```python
from build123d import *

# Parameters (mm, degrees)
F0_R     = 28.3
F0_R_2   = 26.5
F1_DEPTH = 8
F2_SIZE  = 1.5
F3_SIZE  = 0.5
F4_R     = 29.8
F4_R_2   = 28.3
F5_DEPTH = 4.5
F6_SIZE  = 1.49999
F7_SIZE  = 0.5


# Not quite as in the source:
# - a fillet or chamfer is up to 0.001 mm smaller than in the source, because OpenCascade refuses the exact size


with BuildPart() as f1:
    # F0 (on Top) → F1 (new body)
    with BuildSketch(Plane.XY):
        Circle(F0_R)
        Circle(F0_R_2, mode=Mode.SUBTRACT)
    extrude(amount=F1_DEPTH)

    # F2
    f2_edges = [f1.edges().sort_by_distance(p)[0] for p in [
        (-28.3, 0, 8),
    ]]
    chamfer(f2_edges, length=F2_SIZE)

    # F3
    f3_edges = [f1.edges().sort_by_distance(p)[0] for p in [
        (-26.5, 0, 0),
    ]]
    chamfer(f3_edges, length=F3_SIZE)

    # F4 (on face) → F5 (join)
    with BuildSketch(Plane(origin=(0, 0, 0), x_dir=(1, 0, 0), z_dir=(0, 0, -1))):
        Circle(F4_R)
        Circle(F4_R_2, mode=Mode.SUBTRACT)
    extrude(amount=-F5_DEPTH)

    # F6 (size 1.5 in the source; OpenCascade refuses exactly that, so slightly less here)
    f6_edges = [f1.edges().sort_by_distance(p)[0] for p in [
        (-29.8, 0, 4.5),
    ]]
    chamfer(f6_edges, length=F6_SIZE)

    # F7
    f7_edges = [f1.edges().sort_by_distance(p)[0] for p in [
        (-29.8, 0, 0),
    ]]
    chamfer(f7_edges, length=F7_SIZE)


solid = f1.part
```
The listing builds one solid part. Answer for the finished solid, in the listing's coordinates (mm). Round coordinates to 2 decimals unless told otherwise and drop trailing zeros. Write each loop counter-clockwise with the first axis right and the second up, starting at its lowest first coordinate (ties: lowest second). Pieces come first, ordered by that corner, then holes. Notation, with made-up numbers: (0.5, 21) -> (23.5, 21) arc R34 ccw to (23.5, 53) -> close; hole circle Ø7 at (12.5, -33.5). An arc over 180 degrees is marked (long way). Use CSV: the item, a comma, the result in double quotes. Start each with the question number.
(1) Section C-C on z = 3.75 is taken. Give the vertices of the cut face in (x, y), then the cut area to 3 significant figures.
(2) Consider L1, parallel to Y at x = 0, z = 3; L2, parallel to Y at x = 0, z = 5.25; L3, parallel to X at y = -14.5, z = 2.75. Determine where each line is inside the solid, lowest interval first. Write a range as from..to.
(3) Each of these flat-tipped pins is pushed along its axis until it touches: pin 1 (1.5 mm diameter, centred on y = 8.5, z = 3, fed in from -X); pin 2 (2 mm diameter, centred on y = -8, z = 6, fed in from -X); pin 3 (1 mm diameter, centred on y = 16, z = 2.5, fed in from -X). Where does it stop, or does it pass through?
(4) The mould has two halves that part along Y. Classify faces 1 (the face through (14.246, 22.345, 4.198)), 2 (the face through (13, 24, 0)), 3 (the face through (28.424, -8.951, 1.733)): released by +Y, released by -Y, zero draft, split by the parting line, or undercut.
A:
1,outline,"circle Ø58.1 at (0, 0); hole circle Ø53 at (0, 0)"
1,area,"445 mm²"
2,L1,"y = -29.8..-26.5, 26.5..29.8"
2,L2,"y = -28.3..-26.5, 26.5..28.3"
2,L3,"x = -26.03..-22.18, 22.18..26.03"
3,pin 1,"stops at x = -28.77"
3,pin 2,"stops at x = -27.42"
3,pin 3,"stops at x = -25.45"
4,face 1,"undercut"
4,face 2,"zero draft"
4,face 3,"split by the parting line"
